Autodesk Inventor part; units mm, degrees
ref_plane "YZ Plane" through (0, 0, 0) normal (1, 0, 0) x (0, 1, 0)
ref_plane "XZ Plane" through (0, 0, 0) normal (0, 1, 0) x (-1, 0, 0)
ref_plane "XY Plane" through (0, 0, 0) normal (0, 0, 1) x (1, 0, 0)
sketch "Sketch1" plane through (0, 0, 0) normal (1, 0, 0) x (0, 1, 0)
  line L0 (7.5, 15) -> (-7.5, 15)
  line L1 (-7.5, 15) -> (-7.5, -15)
  line L2 (-7.5, -15) -> (7.5, -15)
  line L3 (7.5, -15) -> (7.5, 15)
  point P0 (0, 0)
  dimension "d0" = 30
  dimension "d1" = 15
  dimension "d2" = 7.5
  dimension "d3" = 15
extrude "Extrusion1" add sketch "Sketch1" along normal blind 1
sketch "Sketch2" plane through (0, 7.5, 15) normal (0, 1, 0) x (1, 0, 0)
  circle A0 centre (0.5, 3.3701) radius 0.25
  circle A1 centre (0.5, 29.0879) radius 0.25
  line L0 (0, 30) -> (0, 0)
  point P0 (0, 15)
  dimension "d6" = 0.5
  dimension "d7" = 0.5
  dimension "d8" = 0.5
  dimension "d9" = 0.5
extrude "Extrusion2" cut sketch "Sketch2" against normal blind 20
sketch "Sketch3" plane through (1, 0, 0) normal (1, 0, 0) x (0, 0, -1)
  line L0 (15, 7.5) -> (-15, 0)
  line L1 (-15, 7.5) -> (-15, -7.5)
  line L2 (-15, -7.5) -> (15, -7.5)
  line L3 (15, -7.5) -> (-15, 0)
  point P0 (0, 0)
extrude "Extrusion3" cut sketch "Sketch3" against normal blind 20
sketch "Sketch4" plane through (1, 0, 0) normal (1, 0, 0) x (0, 0, -1)
  line L0 (-15, 0) -> (15, -7.5)
  line L1 (15, 7.5) -> (-15, 0)
  line L2 (-15, 7.5) -> (-15, 0)
  line L3 (-15, 0) -> (-15, 7.5)
  line L4 (-15, 7.5) -> (15, 7.5)
  point P0 (0, 0)
extrude "Extrusion4" cut sketch "Sketch4" against normal blind 20
fillet "Fillet1" radius 0.5 3 edges at (0.5, 0, 15) (0.5, 7.5, -15) (0.5, -7.5, -15)
sketch "Sketch5" plane through (0, 0, 0) normal (-1, 0, 0) x (0, 0, 1)
  line L0 (-15, -6.8596) -> (-15, 6.8596)
  line L1 (-15, -4) -> (-11, -4)
  line L2 (-11, -4) -> (-11, 4)
  line L3 (-11, 4) -> (-15, 4)
  line L4 (-15, 4) -> (-15, -4)
  line L5 (-14.5, -3.5) -> (-11.5, -3.5)
  line L6 (-11.5, -3.5) -> (-11.5, 3.5)
  line L7 (-11.5, 3.5) -> (-14.5, 3.5)
  line L8 (-14.5, 3.5) -> (-14.5, -3.5)
  point P0 (0, 0)
  dimension "d17" = 8
  dimension "d18" = 4
  dimension "d19" = 4
  dimension "d20" = 7
  dimension "d21" = 3
  dimension "d22" = 0.5
  dimension "d23" = 0.5
extrude "Extrusion5" add sketch "Sketch5" along normal blind 5 contours L0 L3 L2 L1 | L8 L7 L6 L5
sketch "Sketch6" plane through (-5, 0, 0) normal (-1, 0, 0) x (0, 0, 1)
  line L0 (-11.5, -3.5) -> (-14.5, -3.5)
  line L1 (-14.5, -3.5) -> (-14.5, 3.5)
  line L2 (-14.5, 3.5) -> (-11.5, 3.5)
  line L3 (-11.5, 3.5) -> (-11.5, -3.5)
  line L4 (-11, -4) -> (-11, 4)
  line L5 (-15, -4) -> (-11, -4)
  point P0 (0, 0)
  dimension "d26" = 7
  dimension "d27" = 3
  dimension "d28" = 0.5
  dimension "d29" = 0.5
extrude "Extrusion6" cut sketch "Sketch6" against normal blind 5
equation "\"BendRadius\" = Thickness"
equation "\"BendReliefWidth\" = Thickness"
equation "\"BendReliefDepth\" = 0.5 * Thickness"
equation "\"CornerReliefSize\" = 4 * Thickness"
equation "\"MinimumRemnant\" = 2 * Thickness"
equation "\"TransitionRadius\" = BendRadius"
equation "\"JacobiRadiusSize\" = BendRadius"
equation "\"GapSize\" = Thickness"
properties part number "ت مهمه 3"
Source: CAD feature listing. Evaluate the final solid. Frame: model axes, mm. A direction names the side the tool comes from. Coordinates: 2 decimals unless noted, no trailing zeros. Loops run counter-clockwise (first coordinate to the right, second up) from the corner with the lowest first, then second, coordinate; pieces in that order, holes last. Notation, with made-up numbers: (-37.75, 84) -> (8.25, 84) arc R22 ccw to (8.25, 92) -> close; hole circle Ø10 at (-0.5, 28). An arc over 180 degrees is marked (long way). Answer in a Markdown table with one row per item. Add a question column.
Q1. Ray query, line 1 along Y through (x, z) = (-3.95, -12); line 2 along Z through (x, y) = (-4.05, -2.25); line 3 along Z through (x, y) = (0.5, -0.25). Return the intervals inside material, ascending.
Q2. Pull-direction query (Y, two-part tool) for faces 1 (the face through (-2, 0, -11)), 2 (the face through (-2, -4, -13)), 3 (the face through (-3, -3.5, -13)); classes: pulls with the +Y half, pulls with the -Y half, needs draft (parallel to the pull), parting line crosses it, or undercut.
Q3. Reachability of faces 4 (the face through (-3, 0, -11.5)), 5 (the face through (-5, 0.3, -14.8)), 6 (the face through (-2, 4, -13)) from +Z, -Z, +X, -X, +Y, -Y: full face, straight path, thin tool, end or side. Return the list, or none.
Q4. Section D-D on y = -1.5. Return the cut outline in (x, z), and give its area (3 significant figures).
Q5. Section B-B on y = 2.75. Return the cut outline in (x, z), and give its area (3 significant figures).
Q6. Section A-A on x = -2.05. Return the cut outline in (y, z).
Q7. Contact query for flat-ended pins moving along their axis: pin 1 Ø2 at (x, z) = (-3, -13.5) entering from -Y; pin 2 Ø2.5 at (y, z) = (-1.5, -13) entering from -X; pin 3 Ø2 at (x, z) = (-1.5, -12.5) entering from +Y. Output: stop coordinate, or through.
Q8. Section C-C on z = 1.25. Return the cut outline in (x, y), and give its area (4 significant figures).
Computed values:
| question | item | result |
|---|---|---|
| 1 | line 1 | y = -4 to -3.5, 3.5 to 4 |
| 1 | line 2 | z = -15 to -14.5, -11.5 to -11 |
| 1 | line 3 | z = -15 to -14.34, -13.84 to 11.38, 11.88 to 13.37 |
| 2 | face 1 | needs draft |
| 2 | face 2 | pulls with the -Y half |
| 2 | face 3 | undercut |
| 3 | face 4 | -X |
| 3 | face 5 | +Z, -Z, -X, +Y, -Y |
| 3 | face 6 | +Z, -Z, -X, +Y |
| 4 | outline | (-5, -15) -> (1, -15) -> (1, 9) -> (0, 9) -> (0, -11) -> (-5, -11) -> (-5, -11.5) -> (0, -11.5) -> (0, -14.5) -> (-5, -14.5) -> close; hole circle Ø0.5 at (0.5, -14.09) |
| 4 | area | 28.8 mm^2 |
| 5 | outline | (-5, -15) -> (1, -15) -> (1, 4) -> (0, 4) -> (0, -11) -> (-5, -11) -> (-5, -11.5) -> (0, -11.5) -> (0, -14.5) -> (-5, -14.5) -> close; hole circle Ø0.5 at (0.5, -14.09) |
| 5 | area | 23.8 mm^2 |
| 6 | outline | (-4, -15) -> (4, -15) -> (4, -11) -> (-4, -11) -> close; hole (-3.5, -14.5) -> (3.5, -14.5) -> (3.5, -11.5) -> (-3.5, -11.5) -> close |
| 7 | pin 1 | stops at y = -4 |
| 7 | pin 2 | stops at x = 0 |
| 7 | pin 3 | stops at y = 4 |
| 8 | outline | (0, -3.44) -> (1, -3.44) -> (1, 3.44) -> (0, 3.44) -> close |
| 8 | area | 6.875 mm^2 |
